Here's the drawing with two shaded views (mm, measured from the low corner). I have some questions. A direction names the side the tool comes from. Coordinates: 2 decimals unless noted, no trailing zeros. Order: outer loops, then holes, each group sorted by start corner. A loop starts at its lowest first (then second) coordinate and runs counter-clockwise, first axis right, second up. Notation, with made-up numbers: (79, 14) - (125, 14) arc R14 cw to (125, 29) - close; hole circle Ø11 at (39, -30). An arc over 180 degrees is marked (long way). Answer as a JSON object with one key per item and string values. Group by question number.
(1) Imagine slicing it at D-D, the plane y = 27. Write out the boundary of the cut face in (x, z), and give its area (3 significant figures).
(2) We'd pull the mould along Y, two halves only. Please class the marked faces 1, 2 and 3: pulls with the +Y half, pulls with the -Y half, needs draft (parallel to the pull), parting line crosses it, or undercut.
(3) Will these pins go through, and if not, where does the flat tip stop? P1, Ø1.5, axis at y = 23, z = 4.5, coming from the +X side; P2, Ø3, axis at y = 37, z = 1.5, coming from the +X side.
(4) Imagine slicing it at B-B, the plane x = 34. Write out the boundary of the cut face in (y, z), and give its area (3 significant figures).
(5) Imagine slicing it at C-C, the plane z = 2.75. Write out the boundary of the cut face in (x, y) (3 decimals).
(6) Which directions (+Z, -Z, +X, -X, +Y, -Y) give clear straight access to the entire face, cutting with the end or side of a thin tool? Please do the marked faces 4 and 5.
(7) Please list where these lines run through material, in increasing order: probe 1 along Y at (x, z) = (23, 5) (3 decimals); probe 2 along Y at (x, z) = (36.5, 0.5).
(8) Imagine slicing it at A-A, the plane x = 23. Write out the boundary of the cut face in (y, z) (3 decimals), and give its area (3 significant figures).
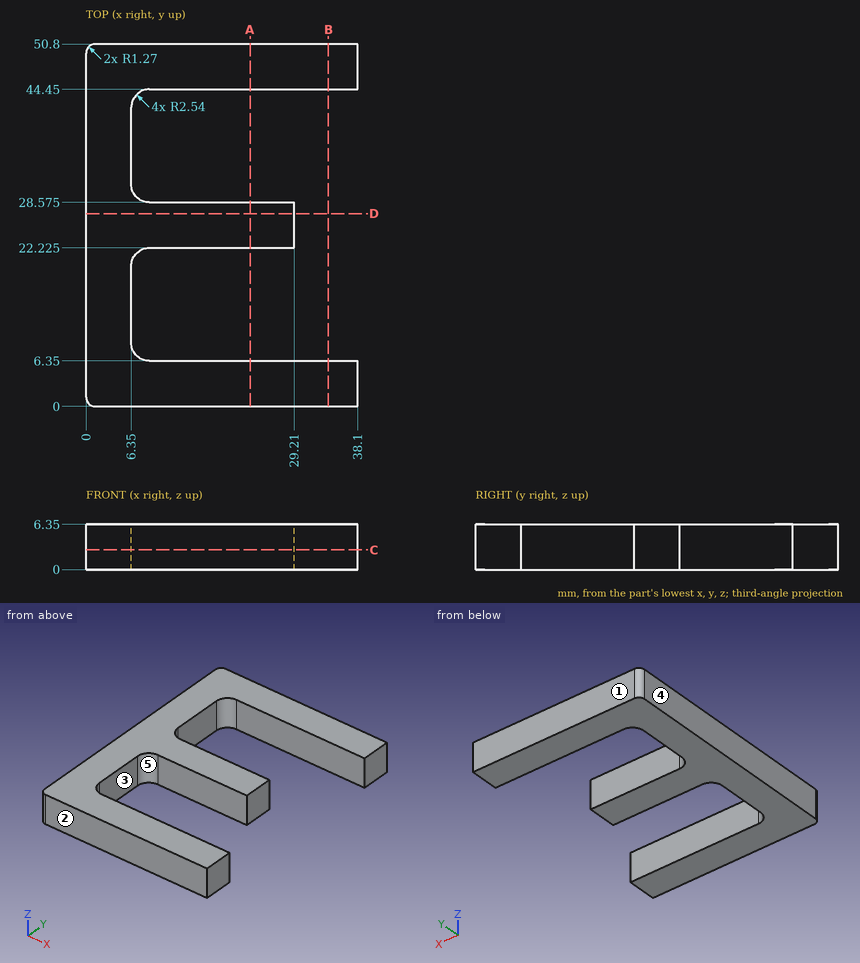
Result set:
{
 "1": {"outline": "(0, 0) - (29.21, 0) - (29.21, 6.35) - (0, 6.35) - close", "area": "185 mm^2"},
 "2": {"face 1": "pulls with the +Y half", "face 2": "pulls with the -Y half", "face 3": "undercut"},
 "3": {"P1": "stops at x = 29.21", "P2": "stops at x = 6.35"},
 "4": {"outline": "(0, 0) - (6.35, 0) - (6.35, 6.35) - (0, 6.35) - close; (44.45, 0) - (50.8, 0) - (50.8, 6.35) - (44.45, 6.35) - close", "area": "80.6 mm^2"},
 "5": {"outline": "(0, 1.27) arc R1.27 ccw to (1.27, 0) - (38.1, 0) - (38.1, 6.35) - (8.89, 6.35) arc R2.54 cw to (6.35, 8.89) - (6.35, 19.685) arc R2.54 cw to (8.89, 22.225) - (29.21, 22.225) - (29.21, 28.575) - (8.89, 28.575) arc R2.54 cw to (6.35, 31.115) - (6.35, 41.91) arc R2.54 cw to (8.89, 44.45) - (38.1, 44.45) - (38.1, 50.8) - (1.27, 50.8) arc R1.27 ccw to (0, 49.53) - close"},
 "6": {"face 4": "+Z, -Z, -X, +Y, -Y", "face 5": "+Z, -Z, +X"},
 "7": {"probe 1": "y = 0 to 6.35, 22.225 to 28.575, 44.45 to 50.8", "probe 2": "y = 0 to 6.35, 44.45 to 50.8"},
 "8": {"outline": "(0, 0) - (6.35, 0) - (6.35, 6.35) - (0, 6.35) - close; (22.225, 0) - (28.575, 0) - (28.575, 6.35) - (22.225, 6.35) - close; (44.45, 0) - (50.8, 0) - (50.8, 6.35) - (44.45, 6.35) - close", "area": "121 mm^2"}
}
